from build123d import *

# Parameters (mm, degrees)
SKETCH1_R           = 17.375
BOSS_EXTRUDE1_DEPTH = 17.7
SKETCH7_R           = 13.545
CUT_EXTRUDE4_DEPTH  = 8
SKETCH10_R          = 3.485
BOSS_EXTRUDE3_DEPTH = 4
SKETCH11_R          = 1.625
CUT_EXTRUDE5_DEPTH  = 13.7


with BuildPart() as part:
    # Sketch1 → Boss-Extrude1 (new body)
    with BuildSketch(Plane(origin=(0, 0, 0), x_dir=(1, 0, 0), z_dir=(0, 1, 0))):
        Circle(SKETCH1_R)
    extrude(amount=BOSS_EXTRUDE1_DEPTH)

    # Sketch7 → Cut-Extrude4 (cut)
    with BuildSketch(Plane.XZ):
        Circle(SKETCH7_R)
    extrude(amount=-CUT_EXTRUDE4_DEPTH, mode=Mode.SUBTRACT)

    # Sketch10 → Boss-Extrude3 (add)
    with BuildSketch(Plane.XZ.offset(-8)):
        Circle(SKETCH10_R)
    extrude(amount=BOSS_EXTRUDE3_DEPTH)

    # Sketch11 → Cut-Extrude5 (cut)
    with BuildSketch(Plane.XZ.offset(-4)):
        Circle(SKETCH11_R)
    extrude(amount=-CUT_EXTRUDE5_DEPTH, mode=Mode.SUBTRACT)


solid = part.part
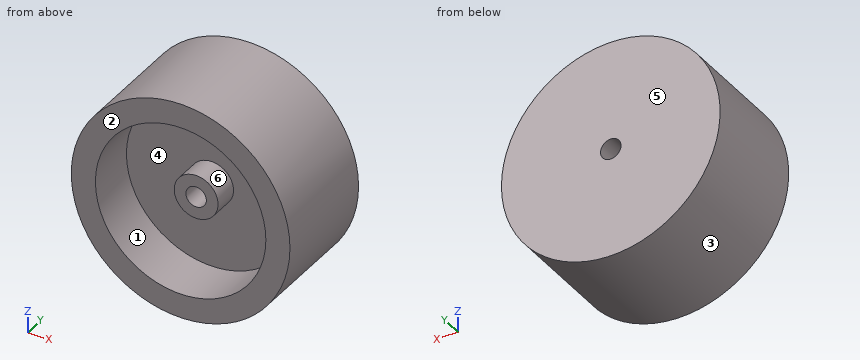
Design review of the part built by this model. Coordinates are the model's own, in mm. Face numbers are marked on the shaded views. A direction names the side the tool comes from. Round coordinates to 2 decimals unless told otherwise and drop trailing zeros. Order: outer loops, then holes, each group sorted by start corner. A loop starts at its lowest first (then second) coordinate and runs counter-clockwise, first axis right, second up.
1) For L1, parallel to Z at x = 2, y = 5.25; L2, parallel to Z at x = 0, y = 6.25 (3 decimals); L3, parallel to Z at x = 0, y = 2 (3 decimals), list the stretches that pass through material, from the lowest coordinate up.
The answers:
L1: z = -17.26 to -13.4, -2.85 to 2.85, 13.4 to 17.26
L2: z = -17.375 to -13.545, -3.485 to -1.625, 1.625 to 3.485, 13.545 to 17.375
L3: z = -17.375 to -13.545, 13.545 to 17.375
2) Draft analysis for pull direction X (two halves, no side actions). For the marked faces 1, 2, 3 and 4, state which applies: released by +X, released by -X, zero draft, split by the parting line, or undercut.
The answers:
face 1: undercut
face 2: zero draft
face 3: split by the parting line
face 4: undercut
3) Clearance check with flat-ended pins moving along their axes: pin 1 Ø1.5 at (x, y) = (-9, 6) entering from -Z; pin 2 Ø6 at (x, z) = (-8.5, -4.5) entering from -Y; pin 3 Ø1.5 at (y, z) = (14.5, 12.5) entering from -X. State where each tip first meets the part, or that it passes through.
The answers:
pin 1: stops at z = -15.29
pin 2: stops at y = 8
pin 3: stops at x = -12.8
4) Consider section B-B (x = 0). State the section outline as (y, z) points (3 decimals), plus the area to 3 significant figures.
The answers:
outline: (0, -17.375) - (17.7, -17.375) - (17.7, -1.625) - (4, -1.625) - (4, -3.485) - (8, -3.485) - (8, -13.545) - (0, -13.545) - close; (0, 13.545) - (8, 13.545) - (8, 3.485) - (4, 3.485) - (4, 1.625) - (17.7, 1.625) - (17.7, 17.375) - (0, 17.375) - close
area: 382 mm2
5) Machinability: for the marked faces 5 and 6, which of the approach directions +Z, -Z, +X, -X, +Y, -Y give a long, thin tool a straight path to every point of the face, cutting with its end or side? Answer none if there is none.
The answers:
face 5: +Z, -Z, +X, -X, +Y
face 6: -Y
6) Consider section C-C (y = 5.75). State the section outline as (x, z) points (3 decimals), plus the area to 3 significant figures.
The answers:
outline: circle Ø34.75 at (0, 0); circle Ø6.97 at (0, 0); hole circle Ø27.09 at (0, 0); hole circle Ø3.25 at (0, 0)
area: 402 mm2
7) Consider section A-A (z = 0). State the section outline as (x, y) points (3 decimals), plus the area to 3 significant figures.
The answers:
outline: (-17.375, 0) - (-13.545, 0) - (-13.545, 8) - (-3.485, 8) - (-3.485, 4) - (-1.625, 4) - (-1.625, 17.7) - (-17.375, 17.7) - close; (1.625, 4) - (3.485, 4) - (3.485, 8) - (13.545, 8) - (13.545, 0) - (17.375, 0) - (17.375, 17.7) - (1.625, 17.7) - close
area: 382 mm2
8) Consider section D-D (y = 3.5). State the section outline as (x, z) points (3 decimals).
The answers:
outline: circle Ø34.75 at (0, 0); hole circle Ø27.09 at (0, 0)
